Geometry check sheet. Reference: the model listing, model coordinates, mm. Face numbers are marked on the shaded views. A direction names the side the tool comes from. Coordinates: 2 decimals unless noted, no trailing zeros. Write each loop counter-clockwise with the first axis right and the second up, starting at its lowest first coordinate (ties: lowest second). Pieces come first, ordered by that corner, then holes. Notation, with made-up numbers: M -4.75,73.5 L 49.25,73.5 A27 ccw 49.25,103.5 Z; hole C 71.25,-7 d8. An arc over 180 degrees is marked long. Write each question's results on one line, items separated by ' | '.
```python
from build123d import *

# Parameters (mm, degrees)
F0_W        = 50.8
F0_H        = 19.05
F1_DEPTH    = 44.45
F2_W        = 3.81
F2_H        = 6.35
F3_DEPTH    = 5.08
F4_R        = 1.0795
F5_DEPTH    = 1.27
F6_R        = 1.0795
F7_DEPTH    = 1.27
F8_T        = 1.27
F8_T3_DEPTH = 6.35
F8_T5_DEPTH = 7.62
F8_T7_DEPTH = 8.89
F9_DEPTH    = 2.54


# Not quite as in the source:
# - a shell that OpenCascade refuses in one call is made with other operations: the cavity is built on its own and cut out


with BuildPart() as f1:
    # F0 (on Top) → F1 (new body)
    with BuildSketch(Plane.XY):
        Rectangle(F0_W, F0_H)
    extrude(amount=F1_DEPTH)

    # F2 (on face) → F3 (cut)
    with BuildSketch(Plane(origin=(0, 0, 0), x_dir=(1, 0, 0), z_dir=(0, 0, -1))):
        with Locations((-23.495, 0)):
            Rectangle(F2_W, F2_H)
    extrude(amount=-F3_DEPTH, mode=Mode.SUBTRACT)

    # F4 (on face) → F5 (cut)
    with BuildSketch(Plane.XZ.offset(-3.175)):
        with Locations((-23.495, 2.54)):
            Circle(F4_R)
    extrude(amount=-F5_DEPTH, mode=Mode.SUBTRACT)

    # F6 (on face) → F7 (cut)
    with BuildSketch(Plane(origin=(0, -3.175, 0), x_dir=(-1, 0, 0), z_dir=(0, 1, 0))):
        with Locations((23.495, 2.54)):
            Circle(F6_R)
    extrude(amount=-F7_DEPTH, mode=Mode.SUBTRACT)

    # F8: shell of thickness 1.27, made by hand


with BuildPart() as f8_core1:
    # F8_t2: copy of F1
    add(f1.part)

    # the walls: a layer under each face that stays
    f8_faces = [f8_core1.faces().sort_by_distance(p)[0] for p in [
        (0, -9.525, 22.225),
        (-25.4, 0, 22.225),
        (25.4, 0, 22.225),
        (0, 0, 44.45),
        (-24.765, 3.175, 4.2333333333),
        (-23.495, 0, 5.08),
        (-22.225, -3.175, 4.2333333333),
        (0, 9.525, 22.225),
        (-21.59, 0, 2.54),
        (-24.5745, 3.81, 2.54),
        (-22.4155, -3.81, 2.54),
        (-23.495, 4.445, 2.54),
        (-23.495, -4.445, 2.54),
    ]]
    thicken(f8_faces, amount=-F8_T, mode=Mode.SUBTRACT)

    # F8_s4 → F8_t3 (cut)
    with BuildSketch(Plane.YZ.offset(-26.67)):
        Polygon((3.1623, 5.0673), (4.445, 5.08), (4.445, 6.35), (3.175, 6.35), align=None)
        Polygon((-3.1623, 5.0673), (-3.175, 6.35), (-4.445, 6.35), (-4.445, 5.08), align=None)
    extrude(amount=F8_T3_DEPTH, mode=Mode.SUBTRACT)

    # F8_s6 → F8_t5 (cut)
    with BuildSketch(Plane.XY.offset(-1.27)):
        Polygon((-21.6027, 3.1623), (-21.59, 4.445), (-20.32, 4.445), (-20.32, 3.175), align=None)
        Polygon((-21.6027, -3.1623), (-21.59, -4.445), (-20.32, -4.445), (-20.32, -3.175), align=None)
    extrude(amount=F8_T5_DEPTH, mode=Mode.SUBTRACT)

    # F8_s8 → F8_t7 (cut)
    with BuildSketch(Plane.XZ.offset(-4.445)):
        Polygon((-21.6027, 5.0673), (-21.59, 6.35), (-20.32, 6.35), (-20.32, 5.08), align=None)
    extrude(amount=F8_T7_DEPTH, mode=Mode.SUBTRACT)

    # F8_s9 → F8_t10 (revolve, cut)
    with BuildSketch(Plane.XY.offset(2.54)):
        Polygon((-22.4282, 4.4323), (-21.1455, 4.445), (-21.1455, 5.715), (-22.4155, 5.715), align=None)
    revolve(axis=Axis((-23.495, 4.445, 2.54), (0, -1, 0)), mode=Mode.SUBTRACT)

    # F8_s11 → F8_t12 (revolve, cut)
    with BuildSketch(Plane.XY.offset(2.54)):
        Polygon((-24.5618, -4.4323), (-25.8445, -4.445), (-25.8445, -5.715), (-24.5745, -5.715), align=None)
    revolve(axis=Axis((-23.495, -4.445, 2.54), (0, 1, 0)), mode=Mode.SUBTRACT)


with BuildPart() as f1_1:
    add(f1.part)

    # what is left inside the walls is the cavity
    f8_cavity = [f8_core1.part.solids().sort_by_distance(p)[0] for p in [
        (0, -8.2423, 28.786667),
    ]]
    add(f8_cavity, mode=Mode.SUBTRACT)

    # F9 (add): a face of the model
    f9_faces = [f1_1.faces().sort_by_distance(p)[0] for p in [
        (-24.13, 0, 23.5412296588),
    ]]
    extrude(f9_faces, amount=F9_DEPTH)


solid = f1_1.part
```
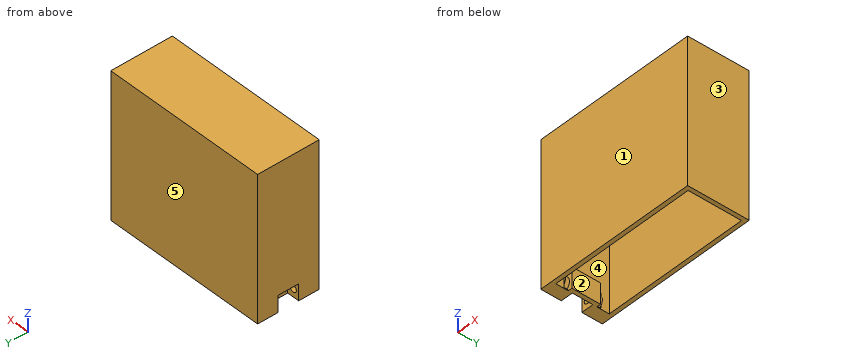
Q1. Sectioned sample at B-B on y = 0.25. Record the cut outline in (x, z), and give its area (3 significant figures).
Geometry check:
outline: M -25.4,5.08 L -21.59,5.08 L -21.59,0 L -20.32,0 L -20.32,6.35 L -21.59,6.35 L -21.59,43.18 L 24.13,43.18 L 24.13,0 L 25.4,0 L 25.4,44.45 L -25.4,44.45 Z | area: 273 mm2
Q2. Sectioned sample at C-C on x = 4. Record the cut outline in (y, z) (3 decimals).
Geometry check:
outline: M -9.525,0 L -8.255,0 L -8.255,43.18 L 8.255,43.18 L 8.255,0 L 9.525,0 L 9.525,44.45 L -9.525,44.45 Z
Q3. Mould release check, pull along X, two halves, no side actions. Record for the marked faces 3, 4 and 5: pulls with the +X half, pulls with the -X half, needs draft (parallel to the pull), parting line crosses it, or undercut.
Geometry check:
face 3: pulls with the +X half | face 4: undercut | face 5: needs draft
Q4. Sectioned sample at D-D on z = 13.5. Record the cut outline in (x, y) (3 decimals).
Geometry check:
outline: M -25.4,-9.525 L 25.4,-9.525 L 25.4,9.525 L -25.4,9.525 Z; hole M -21.59,-8.255 L 24.13,-8.255 L 24.13,8.255 L -21.59,8.255 Z
Q5. Depth check by flat-ended pin: P1, Ø4, axis at x = 4.5, y = 1.5, coming from the -Z side. Enter the tip coordinate at first touch or a pass-through.
Geometry check:
P1: stops at z = 43.18
Q6. Scan lines: probe 1 along Y at (x, z) = (-18, 14.5) (3 decimals); probe 2 along X at (y, z) = (4.25, 27.5); probe 3 along Z at (x, y) = (20, 4.25). Record each from-to range of solid material in increasing order.
Geometry check:
probe 1: y = -9.525 to -8.255, 8.255 to 9.525 | probe 2: x = -25.4 to -21.59, 24.13 to 25.4 | probe 3: z = 43.18 to 44.45
Q7. Access from +Z, -Z, +X, -X, +Y, -Y to the whole of each face (thin tool, end or side, straight path). Record for the marked faces 1 and 2.
Geometry check:
face 1: +Z, -Z, +X, -X, -Y | face 2: -Z
Q8. Sectioned sample at A-A on z = 2.54. Record the cut outline in (x, y) (1 decimal), and give its area (3 significant figures).
Geometry check:
outline: M -25.4,-9.5 L 25.4,-9.5 L 25.4,9.5 L -25.4,9.5 L -25.4,3.2 L -24.6,3.2 L -24.6,4.4 L -22.4,4.4 L -22.4,3.2 L -21.6,3.2 L -21.6,-3.2 L -22.4,-3.2 L -22.4,-4.4 L -24.6,-4.4 L -24.6,-3.2 L -25.4,-3.2 Z; hole M -21.6,-8.3 L 24.1,-8.3 L 24.1,8.3 L -21.6,8.3 L -21.6,5.7 L -21.1,5.7 L -21.1,4.4 L -20.3,4.4 L -20.3,-4.4 L -21.1,-4.4 L -21.1,-5.7 L -21.6,-5.7 Z | area: 196 mm2
